Geometry: final body of the model. Coordinates: model frame, mm. Give positions to 0.01 mm unless a question says otherwise; leave off trailing zeros. Order: outer loops, then holes, each group sorted by start corner. A loop starts at its lowest first (then second) coordinate and runs counter-clockwise, first axis right, second up. Notation, with made-up numbers: (71.5, 39) -> (88.5, 39) arc R14 cw to (88.5, 48) -> close; hole circle Ø9 at (-36, 16). An arc over 180 degrees is marked (long way). One line per question, with ' | ' between items.
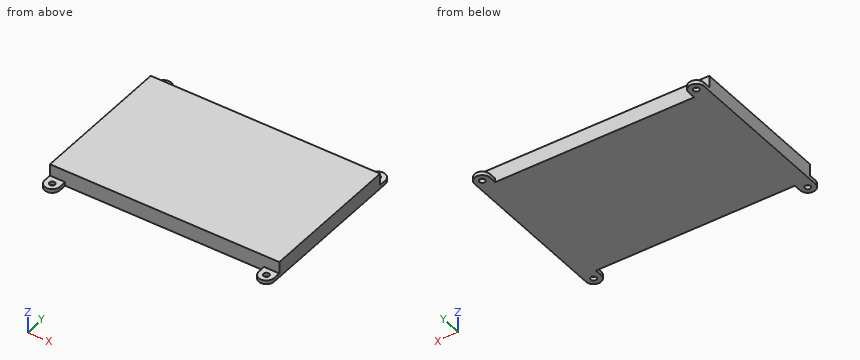
from build123d import *

# Parameters (mm, degrees)
SKETCH1_R           = 4
SKETCH1_R_2         = 1.5
SKETCH1_W           = 120.6
SKETCH1_H           = 76
BOSS_EXTRUDE1_DEPTH = 2
SKETCH4_W           = 120.6
SKETCH4_H           = 76
BOSS_EXTRUDE3_DEPTH = 6.2


with BuildPart() as part:
    # Sketch1 → Boss-Extrude1 (new body)
    # profile 1 of 13: a face of its own
    with BuildSketch(Plane.XY):
        with Locations((-56.3, 42)):
            Circle(SKETCH1_R)
        with Locations((-56.3, 42)):
            Circle(SKETCH1_R_2, mode=Mode.SUBTRACT)
    # profile 2 of 13: a face of its own
    with BuildSketch(Plane.XY):
        with BuildLine():
            Line((-60.3, 42), (-60.3, 38))
            Line((-60.3, 38), (-56.3, 38))
            ThreePointArc((-56.3, 38), (-59.128427125, 39.171572875), (-60.3, 42))
        make_face()
    # profile 3 of 13: a face of its own
    with BuildSketch(Plane.XY):
        with BuildLine():
            ThreePointArc((-52.3, 42), (-53.471572875, 39.171572875), (-56.3, 38))
            Line((-56.3, 38), (-52.3, 38))
            Line((-52.3, 38), (-52.3, 42))
        make_face()
    # profile 4 of 13: a face of its own
    with BuildSketch(Plane.XY):
        Rectangle(SKETCH1_W, SKETCH1_H)
    # profile 5 of 13: a face of its own
    with BuildSketch(Plane.XY):
        with BuildLine():
            ThreePointArc((60.3, 42), (59.128427107, 39.171572857), (56.299999949, 38))
            Line((56.299999949, 38), (60.3, 38))
            Line((60.3, 38), (60.3, 42))
        make_face()
    # profile 6 of 13: a face of its own
    with BuildSketch(Plane.XY):
        with Locations((56.3, 42)):
            Circle(SKETCH1_R)
        with Locations((56.3, 42)):
            Circle(SKETCH1_R_2, mode=Mode.SUBTRACT)
    # profile 7 of 13: a face of its own
    with BuildSketch(Plane.XY):
        with BuildLine():
            Line((52.3, 42), (52.3, 38))
            Line((52.3, 38), (56.299999949, 38))
            ThreePointArc((56.299999949, 38), (53.471572857, 39.171572893), (52.3, 42))
        make_face()
    # profile 8 of 13: a face of its own
    with BuildSketch(Plane.XY):
        with BuildLine():
            Line((-52.3, -38), (-56.3, -38))
            ThreePointArc((-56.3, -38), (-53.471572875, -39.171572875), (-52.3, -42))
            Line((-52.3, -42), (-52.3, -38))
        make_face()
    # profile 9 of 13: a face of its own
    with BuildSketch(Plane.XY):
        with BuildLine():
            Line((-56.3, -38), (-60.3, -38))
            Line((-60.3, -38), (-60.3, -42))
            ThreePointArc((-60.3, -42), (-59.128427125, -39.171572875), (-56.3, -38))
        make_face()
    # profile 10 of 13: a face of its own
    with BuildSketch(Plane.XY):
        with Locations((-56.3, -42)):
            Circle(SKETCH1_R)
        with Locations((-56.3, -42)):
            Circle(SKETCH1_R_2, mode=Mode.SUBTRACT)
    # profile 11 of 13: a face of its own
    with BuildSketch(Plane.XY):
        with BuildLine():
            Line((56.3, -38), (52.3, -38))
            Line((52.3, -38), (52.3, -42))
            ThreePointArc((52.3, -42), (53.471572875, -39.171572875), (56.3, -38))
        make_face()
    # profile 12 of 13: a face of its own
    with BuildSketch(Plane.XY):
        with Locations((56.3, -42)):
            Circle(SKETCH1_R)
        with Locations((56.3, -42)):
            Circle(SKETCH1_R_2, mode=Mode.SUBTRACT)
    # profile 13 of 13: a face of its own
    with BuildSketch(Plane.XY):
        with BuildLine():
            Line((60.3, -38), (56.3, -38))
            ThreePointArc((56.3, -38), (59.128427125, -39.171572875), (60.3, -42))
            Line((60.3, -42), (60.3, -38))
        make_face()
    extrude(amount=BOSS_EXTRUDE1_DEPTH)

    # Sketch4 → Boss-Extrude3 (add)
    with BuildSketch(Plane.XY.offset(2)):
        Rectangle(SKETCH4_W, SKETCH4_H)
    extrude(amount=BOSS_EXTRUDE3_DEPTH)


solid = part.part
1) Section C-C on x = 39.5. Return loops of the section in (y, z).
Check result:
outline: (-38, 0) -> (38, 0) -> (38, 8.2) -> (-38, 8.2) -> close
2) Contact query for flat-ended pins moving along their axis: pin 1 Ø6.5 at (x, y) = (57, 43.5) entering from +Z; pin 2 Ø2.5 at (x, z) = (-26, 4) entering from +Y; pin 3 Ø4 at (x, z) = (35, 6.5) entering from -Y. Output: stop coordinate, or through.
Check result:
pin 1: stops at z = 2 | pin 2: stops at y = 38 | pin 3: stops at y = -38
3) Section B-B on z = 5.5. Return loops of the section in (x, y), plus the area to 3 significant figures.
Check result:
outline: (-60.3, -38) -> (60.3, -38) -> (60.3, 38) -> (-60.3, 38) -> close | area: 9,170 mm^2
4) Section A-A on x = -56.3. Return loops of the section in (y, z), plus the area to 3 significant figures.
Check result:
outline: (-46, 0) -> (-43.5, 0) -> (-43.5, 2) -> (-46, 2) -> close; (-40.5, 0) -> (40.5, 0) -> (40.5, 2) -> (38, 2) -> (38, 8.2) -> (-38, 8.2) -> (-38, 2) -> (-40.5, 2) -> close; (43.5, 0) -> (46, 0) -> (46, 2) -> (43.5, 2) -> close | area: 643 mm^2
5) Material intervals for probe 1 along Y at (x, z) = (56.3, 1.15); probe 2 along Y at (x, z) = (-51, 6), sorted ascending. Write a range as from..to.
Check result:
probe 1: y = -46..-43.5, -40.5..40.5, 43.5..46 | probe 2: y = -38..38
